Input: part model. Units: mm. Frame: model coordinates. Face numbers are marked on the shaded views. A direction names the side the tool comes from. Round coordinates to 2 decimals unless told otherwise and drop trailing zeros. Loops run counter-clockwise (first coordinate to the right, second up) from the corner with the lowest first, then second, coordinate; pieces in that order, holes last. Notation, with made-up numbers: (-12, 66) -> (26, 66) arc R27 ccw to (26, 83) -> close; hole circle Ø5 at (26.25, -35.75). An arc over 180 degrees is marked (long way). Answer as a JSON object with one key per item and string values.
```python
from build123d import *

# Parameters (mm, degrees)
SKETCH2_R           = 2.5
BOSS_EXTRUDE1_DEPTH = 66


with BuildPart() as part:
    # Sketch1 → Revolve1 (revolve)
    with BuildSketch(Plane.XY):
        with BuildLine():
            Line((0, 0), (0, 8.25))
            Line((0, 8.25), (9.5, 8.25))
            Line((9.5, 8.25), (9.5, 9))
            Line((9.5, 9), (39.5, 9))
            ThreePointArc((39.5, 9), (42.338390167, 4.923262843), (43, 0))
            Line((43, 0), (0, 0))
        make_face()
    revolve(axis=Axis((0, 0, 0), (1, 0, 0)))

    # Sketch2 → Boss-Extrude1 (add)
    with BuildSketch(Plane.ZY):
        Circle(SKETCH2_R)
    extrude(amount=-BOSS_EXTRUDE1_DEPTH)


solid = part.part
```
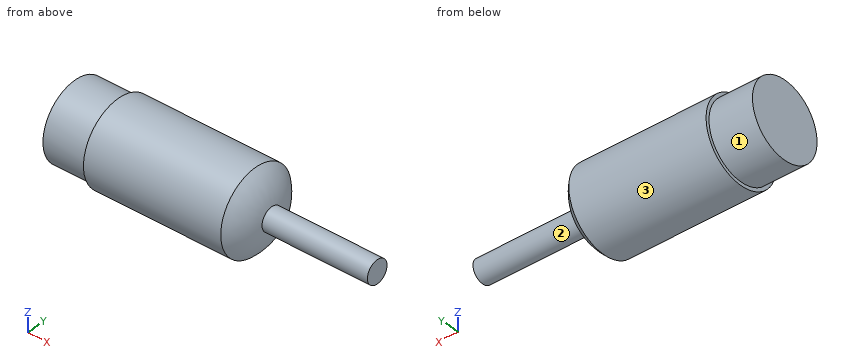
1) Section A-A, the plane x = 18.5. Output: boundary loops of the cut face in (y, z).
Output:
{"outline": "circle Ø18 at (0, 0)"}
2) Contact query for flat-ended pins moving along their axis: P1, Ø4, axis at x = 7.5, y = 7, coming from the -Z side; P2, Ø1.5, axis at x = 41.5, z = -1.5, coming from the -Y side; P3, Ø5, axis at x = 26.5, y = -6.5, coming from the -Z side. Output: stop coordinate, or through.
Output:
{"P1": "stops at z = -6.56", "P2": "stops at y = -7.55", "P3": "stops at z = -8.06"}
3) Reachability of the marked faces 1, 2 and 3 from +Z, -Z, +X, -X, +Y, -Y: full face, straight path, thin tool, end or side. Return the list, or none.
Output:
{"face 1": "-X", "face 2": "+X", "face 3": "+X, -X"}
4) Section B-B, the plane x = 50. Output: boundary loops of the cut face in (y, z), plus the area to 3 significant figures.
Output:
{"outline": "circle Ø5 at (0, 0)", "area": "19.6 mm^2"}
5) Ray query, probe 1 along Y at (x, z) = (33, 0.5); probe 2 along X at (y, z) = (-6.5, -2.25). Return the intervals inside material, ascending.
Output:
{"probe 1": "y = -8.99 to 8.99", "probe 2": "x = 0 to 41.33"}
